from build123d import *

# Parameters (mm, degrees)
BOSS_EXTRUDE1_DEPTH = 3.175
SKETCH4_W           = 6.35
SKETCH4_H           = 3.175
BOSS_EXTRUDE3_DEPTH = 7.62
FILLET2_R           = 1.27
SKETCH8_W           = 6.35
SKETCH8_H           = 6.35
BOSS_EXTRUDE5_DEPTH = 7.62
SKETCH7_R           = 1.627
CUT_EXTRUDE3_DEPTH  = 63.5
FILLET3_R           = 3.175
SKETCH9_R           = 1.627
CUT_EXTRUDE4_DEPTH  = 6.35
CUT_EXTRUDE5_REACH  = 70.976
SKETCH10_R          = 1.627


with BuildPart() as part:
    # Sketch2 → Boss-Extrude1 (new, symmetric)
    with BuildSketch(Plane(origin=(0, 0, 0), x_dir=(0, 0, -1), z_dir=(1, 0, 0))):
        Polygon((-25.4, 26.035), (-25.4, 3.175), (-25.4, -3.175), (-19.05, -3.175), (-19.05, 3.175), (-19.05, 9.525), (-19.05, 24.333522628), (-17.708087105, 26.657783942), (17.708087105, 26.657783942), (19.05, 24.333522628), (19.05, 3.175), (19.05, -3.175), (25.4, -3.175), (25.4, 3.175), (25.4, 26.035), (9.525, 53.53130657), (0, 53.53130657), (-9.525, 53.53130657), align=None)
        Polygon((-14.041912895, 33.007783942), (-5.858825791, 47.18130657), (0, 47.18130657), (5.858825791, 47.18130657), (14.041912895, 33.007783942), align=None, mode=Mode.SUBTRACT)
    extrude(amount=BOSS_EXTRUDE1_DEPTH, both=True)

    # Sketch4 → Boss-Extrude3 (add)
    with BuildSketch(Plane.XZ.offset(-26.657783942)):
        with Locations((0, -4.7625)):
            Rectangle(SKETCH4_W, SKETCH4_H)
        with Locations((0, 4.7625)):
            Rectangle(SKETCH4_W, SKETCH4_H)
    extrude(amount=BOSS_EXTRUDE3_DEPTH)

    # Fillet2
    fillet2_edges = [part.edges().sort_by_distance(p)[0] for p in [
        (3.175, 40.094545256, -9.950369343),
        (3.175, 33.007783942, 0),
        (-3.175, 26.657783942, -12.029043552),
        (-3.175, 25.495653285, 18.379043552),
        (-3.175, 10.579261314, 19.05),
        (-3.175, 11.43, 25.4),
        (-3.175, 39.783153285, 17.4625),
        (-3.175, 39.783153285, -17.4625),
        (3.175, 40.094545256, 9.950369343),
        (-3.175, 11.43, -25.4),
        (-3.175, 10.579261314, -19.05),
        (-3.175, 25.495653285, -18.379043552),
        (-3.175, 40.094545256, 9.950369343),
        (-3.175, 33.007783942, 0),
        (-3.175, 40.094545256, -9.950369343),
        (-3.175, 47.18130657, 0),
        (3.175, 25.495653285, -18.379043552),
        (0, 24.333522628, 19.05),
        (0, -3.175, 19.05),
        (3.175, 10.579261314, -19.05),
        (0, -3.175, 25.4),
        (0, 26.035, 25.4),
        (0, 53.53130657, 9.525),
        (0, 53.53130657, -9.525),
        (0, 26.035, -25.4),
        (0, -3.175, -25.4),
        (0, -3.175, -19.05),
        (0, 24.333522628, -19.05),
        (0, 33.007783942, 14.041912895),
        (0, 33.007783942, -14.041912895),
        (3.175, 11.43, -25.4),
        (3.175, 39.783153285, -17.4625),
        (-3.175, 26.657783942, 12.029043552),
        (3.175, 26.657783942, 12.029043552),
        (3.175, 39.783153285, 17.4625),
        (3.175, 11.43, 25.4),
        (-3.175, 26.657783942, 0),
        (3.175, 26.657783942, 0),
        (3.175, 47.18130657, 0),
        (3.175, 10.579261314, 19.05),
        (3.175, 25.495653285, 18.379043552),
        (3.175, 26.657783942, -12.029043552),
    ]]
    fillet(fillet2_edges, radius=FILLET2_R)

    # Sketch8 → Boss-Extrude5 (add)
    with BuildSketch(Plane(origin=(0, 53.53130657, 0), x_dir=(1, 0, 0), z_dir=(0, 1, 0))):
        Rectangle(SKETCH8_W, SKETCH8_H)
    extrude(amount=BOSS_EXTRUDE5_DEPTH)

    # Sketch7 → Cut-Extrude3 (cut)
    with BuildSketch(Plane(origin=(0, 0, -25.4), x_dir=(-1, 0, 0), z_dir=(0, 0, -1))):
        Circle(SKETCH7_R)
    extrude(amount=-CUT_EXTRUDE3_DEPTH, mode=Mode.SUBTRACT)

    # Fillet3
    # the kernel refuses this fillet: 3.175 mm, written as the material it takes off along each edge
    with BuildSketch(Plane(origin=(0, 0, 25.4), x_dir=(0, -1, 0), z_dir=(-1, 0, 0))) as fillet3_piece_1:
        with BuildLine():
            CenterArc((1.905, -1.27), 1.27, 0, 90)
            Line((3.175, -1.27), (3.175, 0))
            Line((3.175, 0), (1.905, 0))
        make_face()
    revolve(axis=Axis((0, 0, 25.4), (0, 0, 1)), revolution_arc=90, mode=Mode.SUBTRACT)
    with BuildSketch(Plane(origin=(0, 0, 19.05), x_dir=(1, 0, 0), z_dir=(0, 1, 0))) as fillet3_piece_2:
        with BuildLine():
            CenterArc((1.905, -1.27), 1.27, 0, 90)
            Line((3.175, -1.27), (3.175, 0))
            Line((3.175, 0), (1.905, 0))
        make_face()
    revolve(axis=Axis((0, 0, 19.05), (0, 0, -1)), revolution_arc=90, mode=Mode.SUBTRACT)
    with BuildSketch(Plane(origin=(0, 0, 25.4), x_dir=(-1, 0, 0), z_dir=(0, 1, 0))) as fillet3_piece_3:
        with BuildLine():
            CenterArc((1.905, -1.27), 1.27, 0, 90)
            Line((3.175, -1.27), (3.175, 0))
            Line((3.175, 0), (1.905, 0))
        make_face()
    revolve(axis=Axis((0, 0, 25.4), (0, 0, 1)), revolution_arc=90, mode=Mode.SUBTRACT)
    with BuildSketch(Plane(origin=(0, 0, 19.05), x_dir=(0, -1, 0), z_dir=(1, 0, 0))) as fillet3_piece_4:
        with BuildLine():
            CenterArc((1.905, -1.27), 1.27, 0, 90)
            Line((3.175, -1.27), (3.175, 0))
            Line((3.175, 0), (1.905, 0))
        make_face()
    revolve(axis=Axis((0, 0, 19.05), (0, 0, -1)), revolution_arc=90, mode=Mode.SUBTRACT)
    with BuildSketch(Plane(origin=(0, 0, -25.4), x_dir=(1, 0, 0), z_dir=(0, 1, 0))) as fillet3_piece_5:
        with BuildLine():
            CenterArc((1.905, -1.27), 1.27, 0, 90)
            Line((3.175, -1.27), (3.175, 0))
            Line((3.175, 0), (1.905, 0))
        make_face()
    revolve(axis=Axis((0, 0, -25.4), (0, 0, -1)), revolution_arc=90, mode=Mode.SUBTRACT)
    with BuildSketch(Plane(origin=(0, 0, -25.4), x_dir=(0, -1, 0), z_dir=(1, 0, 0))) as fillet3_piece_6:
        with BuildLine():
            CenterArc((1.905, -1.27), 1.27, 0, 90)
            Line((3.175, -1.27), (3.175, 0))
            Line((3.175, 0), (1.905, 0))
        make_face()
    revolve(axis=Axis((0, 0, -25.4), (0, 0, -1)), revolution_arc=90, mode=Mode.SUBTRACT)
    with BuildSketch(Plane(origin=(0, 0, -19.05), x_dir=(0, -1, 0), z_dir=(-1, 0, 0))) as fillet3_piece_7:
        with BuildLine():
            CenterArc((1.905, -1.27), 1.27, 0, 90)
            Line((3.175, -1.27), (3.175, 0))
            Line((3.175, 0), (1.905, 0))
        make_face()
    revolve(axis=Axis((0, 0, -19.05), (0, 0, 1)), revolution_arc=90, mode=Mode.SUBTRACT)
    with BuildSketch(Plane(origin=(0, 0, -19.05), x_dir=(-1, 0, 0), z_dir=(0, 1, 0))) as fillet3_piece_8:
        with BuildLine():
            CenterArc((1.905, -1.27), 1.27, 0, 90)
            Line((3.175, -1.27), (3.175, 0))
            Line((3.175, 0), (1.905, 0))
        make_face()
    revolve(axis=Axis((0, 0, -19.05), (0, 0, 1)), revolution_arc=90, mode=Mode.SUBTRACT)
    with BuildSketch(Plane(origin=(-3.175, 19.037783942, -4.7625), x_dir=(0, 1, 0), z_dir=(0, 0, 1)), Plane(origin=(3.175, 19.037783942, 14.2875), x_dir=(0, 1, 0), z_dir=(0, 0, -1))) as fillet3_piece_9:
        with BuildLine():
            CenterArc((FILLET3_R, -FILLET3_R), FILLET3_R, 90, 90)
            Line((0, -FILLET3_R), (0, 0))
            Line((0, 0), (FILLET3_R, 0))
        make_face()
    extrude(amount=19.05, mode=Mode.SUBTRACT)
    with BuildSketch(Plane(origin=(-3.175, 19.037783942, 4.7625), x_dir=(0, 1, 0), z_dir=(0, 0, -1)), Plane(origin=(3.175, 19.037783942, -14.2875), x_dir=(0, 1, 0), z_dir=(0, 0, 1))) as fillet3_piece_10:
        with BuildLine():
            CenterArc((FILLET3_R, FILLET3_R), FILLET3_R, 180, 90)
            Line((0, FILLET3_R), (0, 0))
            Line((0, 0), (FILLET3_R, 0))
        make_face()
    extrude(amount=19.05, mode=Mode.SUBTRACT)
    with BuildSketch(Plane(origin=(-3.175, 61.15130657, 11.1125), x_dir=(0, -1, 0), z_dir=(0, 0, -1)), Plane(origin=(3.175, 61.15130657, -11.1125), x_dir=(0, -1, 0), z_dir=(0, 0, 1))) as fillet3_piece_11:
        with BuildLine():
            CenterArc((FILLET3_R, -FILLET3_R), FILLET3_R, 90, 90)
            Line((0, -FILLET3_R), (0, 0))
            Line((0, 0), (FILLET3_R, 0))
        make_face()
    extrude(amount=22.225, mode=Mode.SUBTRACT)
    with BuildSketch(Plane(origin=(-3.175, -3.175, 25.4), x_dir=(0, 1, 0), z_dir=(0, 0, -1)), Plane(origin=(-3.175, -3.175, -19.05), x_dir=(0, 1, 0), z_dir=(0, 0, -1))) as fillet3_piece_12:
        with BuildLine():
            CenterArc((FILLET3_R, FILLET3_R), FILLET3_R, 180, 90)
            Line((0, FILLET3_R), (0, 0))
            Line((0, 0), (FILLET3_R, 0))
        make_face()
    extrude(amount=6.35, mode=Mode.SUBTRACT)
    with BuildSketch(Plane(origin=(3.175, -3.175, 25.4), x_dir=(0, 1, 0), z_dir=(0, 0, -1)), Plane(origin=(3.175, -3.175, -19.05), x_dir=(0, 1, 0), z_dir=(0, 0, -1))) as fillet3_piece_13:
        with BuildLine():
            CenterArc((FILLET3_R, -FILLET3_R), FILLET3_R, 90, 90)
            Line((0, -FILLET3_R), (0, 0))
            Line((0, 0), (FILLET3_R, 0))
        make_face()
    extrude(amount=6.35, mode=Mode.SUBTRACT)

    # Sketch9 → Cut-Extrude4 (cut)
    with BuildSketch(Plane.XY.offset(3.175)):
        with Locations((0, 57.97630657)):
            Circle(SKETCH9_R)
    extrude(amount=-CUT_EXTRUDE4_DEPTH, mode=Mode.SUBTRACT)

    # Cut-Extrude5: up to this face of the body (flat: up to its plane)
    cut_extrude5_end = Plane(part.part.faces().sort_by_distance((0, 23.210890681, -6.35))[0])
    # Sketch10 → Cut-Extrude5 (cut, up to the picked face)
    with BuildSketch(Plane.XY.offset(6.35), mode=Mode.PRIVATE) as cut_extrude5_sk1:
        with Locations((0, 22.212783942)):
            Circle(SKETCH10_R)
    cut_extrude5_tool1 = split(extrude(cut_extrude5_sk1.sketch, amount=-CUT_EXTRUDE5_REACH, mode=Mode.PRIVATE), bisect_by=cut_extrude5_end, keep=Keep.BOTH, mode=Mode.PRIVATE)
    add(cut_extrude5_tool1.solids().sort_by(Axis((0, 22.212784, 6.35), (0, 0, -1)))[0], mode=Mode.SUBTRACT)


solid = part.part
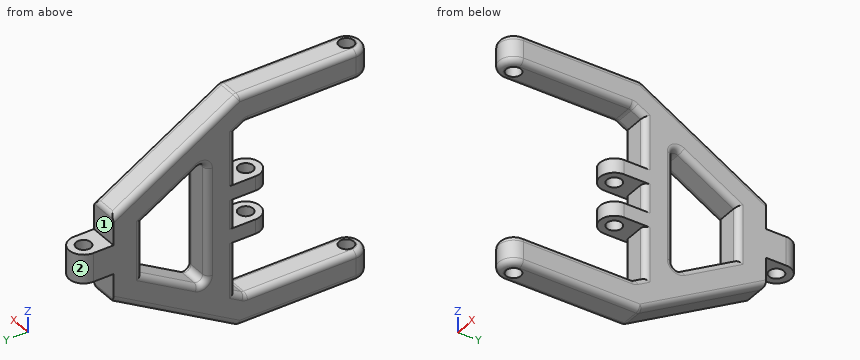
For this review, take the finished solid that the model builds, in its own axes (mm). Face numbers are marked on the shaded views. A direction names the side the tool comes from. Give positions to 0.01 mm unless a question says otherwise; leave off trailing zeros. Order: outer loops, then holes, each group sorted by start corner. A loop starts at its lowest first (then second) coordinate and runs counter-clockwise, first axis right, second up. Notation, with made-up numbers: M 30,33.5 L 35,33.5 A15 ccw 35,53.5 Z; hole C 4,-24.75 d4. An arc over 180 degrees is marked long. Answer in a Markdown table with one row per item. Add a question column.
(1) For the marked faces 1 and 2, list the 3-axis set-ups (+Z, -Z, +X, -X, +Y, -Y) from which the entire face can be reached by the end or side of a thin tool; tool diameter is ignored.
(2) Wall thickness on probe 1 along Y at (x, z) = (0, -3.8); probe 2 along Z at (x, y) = (-1.5, 23.5) (3 decimals); probe 3 along Z at (x, y) = (-0.75, 6.5): over which ranges is each line inside the solid? List them lowest first. Write a range as [from, to].
(3) Consider section C-C on y = 9. State the section outline as (x, z) points (3 decimals).
(4) Consider section A-A on z = -4.5. State the section outline as (x, y) points (3 decimals).
(5) Consider section D-D on z = 1. State the section outline as (x, y) points (3 decimals).
(6) Consider section B-B on x = 0. Give the number of separate pieces and of enclosed holes in the cut face, and give its area (3 significant figures).
(7) For pin 1 (3 mm diameter, centred on x = 0.5, y = 50, fed in from -Z); pin 2 (3 mm diameter, centred on x = -0.5, z = -6.5, fed in from +Y); pin 3 (2 mm diameter, centred on x = 0, z = -15.5, fed in from +Y), all flat-tipped, find the tip position at first contact; note any pin that passes through.
Evaluation:
| question | item | result |
|---|---|---|
| 1 | face 1 | +Z, +X, -X, +Y |
| 1 | face 2 | +Z, -Z, +Y |
| 2 | probe 1 | y = [19.04, 20.59], [23.84, 33.01], [47.18, 53.53] |
| 2 | probe 2 | z = [-25.4, -19.05], [-6.35, -3.175], [3.175, 6.35], [19.05, 25.4] |
| 2 | probe 3 | z = [-25.4, -19.05], [19.05, 25.4] |
| 3 | outline | M -3.175,-24.13 A1.27 ccw -1.905,-25.4 L 1.905,-25.4 A1.27 ccw 3.175,-24.13 L 3.175,-20.32 A1.27 ccw 1.905,-19.05 L -1.905,-19.05 A1.27 ccw -3.175,-20.32 Z; M -3.175,20.32 A1.27 ccw -1.905,19.05 L 1.905,19.05 A1.27 ccw 3.175,20.32 L 3.175,24.13 A1.27 ccw 1.905,25.4 L -1.905,25.4 A1.27 ccw -3.175,24.13 Z |
| 4 | outline | M -3.175,22.213 A3.175 ccw 3.175,22.213 L 3.175,31.738 A1.27 ccw 1.905,33.008 L -1.905,33.008 A1.27 ccw -3.175,31.738 Z; M -3.175,48.451 A1.27 ccw -1.905,47.181 L 1.905,47.181 A1.27 ccw 3.175,48.451 L 3.175,53.531 L -3.175,53.531 Z; hole C 0,22.213 d3.254 |
| 5 | outline | M -3.175,27.928 A1.27 ccw -1.905,26.658 L 1.905,26.658 A1.27 ccw 3.175,27.928 L 3.175,31.738 A1.27 ccw 1.905,33.008 L -1.905,33.008 A1.27 ccw -3.175,31.738 Z; M -3.175,48.451 A1.27 ccw -1.905,47.181 L 1.905,47.181 A1.27 ccw 3.175,48.451 L 3.175,57.976 A3.175 ccw -3.175,57.976 Z; hole C 0,57.976 d3.254 |
| 6 | separate pieces | 6 |
| 6 | enclosed holes | 1 |
| 6 | area | 1,040 mm^2 |
| 7 | pin 1 | stops at z = -12.43 |
| 7 | pin 2 | stops at y = 53.53 |
| 7 | pin 3 | stops at y = 44.91 |
